Work out the finished part from the listing and answer in its coordinate system (mm). A direction names the side the tool comes from. Round coordinates to 2 decimals unless told otherwise and drop trailing zeros. Loops run counter-clockwise (first coordinate to the right, second up) from the corner with the lowest first, then second, coordinate; pieces in that order, holes last.
```python
from build123d import *

# Parameters (mm, degrees)
SKETCH1_W           = 150
SKETCH1_H           = 112
BOSS_EXTRUDE1_DEPTH = 6
SKETCH3_W           = 150
SKETCH3_H           = 6
BOSS_EXTRUDE2_DEPTH = 8
SKETCH4_W           = 150
SKETCH4_H           = 4
BOSS_EXTRUDE3_DEPTH = 8
SKETCH6_W           = 150
SKETCH6_H           = 36
BOSS_EXTRUDE4_DEPTH = 60
CUT_EXTRUDE1_START  = -4
SKETCH7_W           = 150
SKETCH7_H           = 74
CUT_EXTRUDE1_DEPTH  = 4
SKETCH8_W           = 142
SKETCH8_H           = 58
CUT_EXTRUDE2_DEPTH  = 28


with BuildPart() as part:
    # Sketch1 → Boss-Extrude1 (new body)
    with BuildSketch(Plane(origin=(0, 0, 0), x_dir=(1, 0, 0), z_dir=(0, 1, 0))):
        with Locations((0, -6)):
            Rectangle(SKETCH1_W, SKETCH1_H)
    extrude(amount=BOSS_EXTRUDE1_DEPTH)

    # Sketch3 → Boss-Extrude2 (add)
    with BuildSketch(Plane.XY.offset(62)):
        with Locations((0, 3)):
            Rectangle(SKETCH3_W, SKETCH3_H)
    extrude(amount=BOSS_EXTRUDE2_DEPTH)

    # Sketch4 → Boss-Extrude3 (add)
    with BuildSketch(Plane(origin=(0, 0, 0), x_dir=(-1, 0, 0), z_dir=(0, -1, 0))):
        with Locations((0, -68)):
            Rectangle(SKETCH4_W, SKETCH4_H)
    extrude(amount=BOSS_EXTRUDE3_DEPTH)

    # Sketch6 → Boss-Extrude4 (add)
    with BuildSketch(Plane(origin=(0, 6, 0), x_dir=(1, 0, 0), z_dir=(0, 1, 0))):
        with Locations((0, -52)):
            Rectangle(SKETCH6_W, SKETCH6_H)
    extrude(amount=BOSS_EXTRUDE4_DEPTH)

    # Sketch7 → Cut-Extrude1 (cut)
    with BuildSketch(Plane.XY.offset(70).offset(CUT_EXTRUDE1_START)):
        with Locations((0, 29)):
            Rectangle(SKETCH7_W, SKETCH7_H)
    extrude(amount=CUT_EXTRUDE1_DEPTH, mode=Mode.SUBTRACT)

    # Sketch8 → Cut-Extrude2 (cut)
    with BuildSketch(Plane.XY.offset(66)):
        with Locations((0, 33)):
            Rectangle(SKETCH8_W, SKETCH8_H)
    extrude(amount=-CUT_EXTRUDE2_DEPTH, mode=Mode.SUBTRACT)


solid = part.part
```
1. Find section A-A (x = 0). Write down the section's boundary in (y, z), then the cut area to 3 significant figures.
Answer key:
outline: (0, -50) - (6, -50) - (6, 34) - (66, 34) - (66, 66) - (62, 66) - (62, 38) - (4, 38) - (4, 66) - (0, 66) - close
area: 992 mm2
2. Find section C-C (z = -33.5). Write down the section's boundary in (x, y), then the cut area to 3 significant figures.
Answer key:
outline: (-75, 0) - (75, 0) - (75, 6) - (-75, 6) - close
area: 900 mm2
3. Which of the six approach directions +Z, -Z, +X, -X, +Y, -Y give full straight-line access (tool end or side, diameter ignored) to faces 4 (the face through (-1, 62, 52)), 5 (the face through (-1, 66, 50)), 6 (the face through (-1, 36, 34))?
Answer key:
face 4: +Z
face 5: +Z, -Z, +X, -X, +Y
face 6: -Z, +X, -X, +Y
4. Find section B-B (y = 11). Write down the section's boundary in (x, z).
Answer key:
outline: (-75, 34) - (75, 34) - (75, 66) - (71, 66) - (71, 38) - (-71, 38) - (-71, 66) - (-75, 66) - close
5. Consider probe 1 along Y at (x, z) = (-20.5, 50); probe 2 along X at (y, z) = (56.5, 42); probe 3 along Z at (x, y) = (20, 23.5). Determine where each line is inside the solid, lowest interval first.
Answer key:
probe 1: y = 0 to 4, 62 to 66
probe 2: x = -75 to -71, 71 to 75
probe 3: z = 34 to 38
6. Given pin 1 (6 mm diameter, centred on x = -21.5, y = 14.5, fed in from +Z); pin 2 (14 mm diameter, centred on x = 28.5, z = 47, fed in from -Y); pin 3 (1.5 mm diameter, centred on x = 2.5, y = 45, fed in from -Z); pin 4 (25 mm diameter, centred on x = 34, z = 10, fed in from +Y), each flat-ended and moving along its own axis, determine where each tip first touches the part or whether it passes through.
Answer key:
pin 1: stops at z = 38
pin 2: stops at y = 0
pin 3: stops at z = 34
pin 4: stops at y = 6
7. Determine the mould class of faces 1 (the face through (-5.9, 3.8, 66)), 2 (the face through (-75, 25, 35)), 3 (the face through (-1, 33, 38)) for opening direction X: +X half, -X half, draft (parallel to the pull), parting line (faces both ways), or undercut.
Answer key:
face 1: draft
face 2: -X half
face 3: undercut
